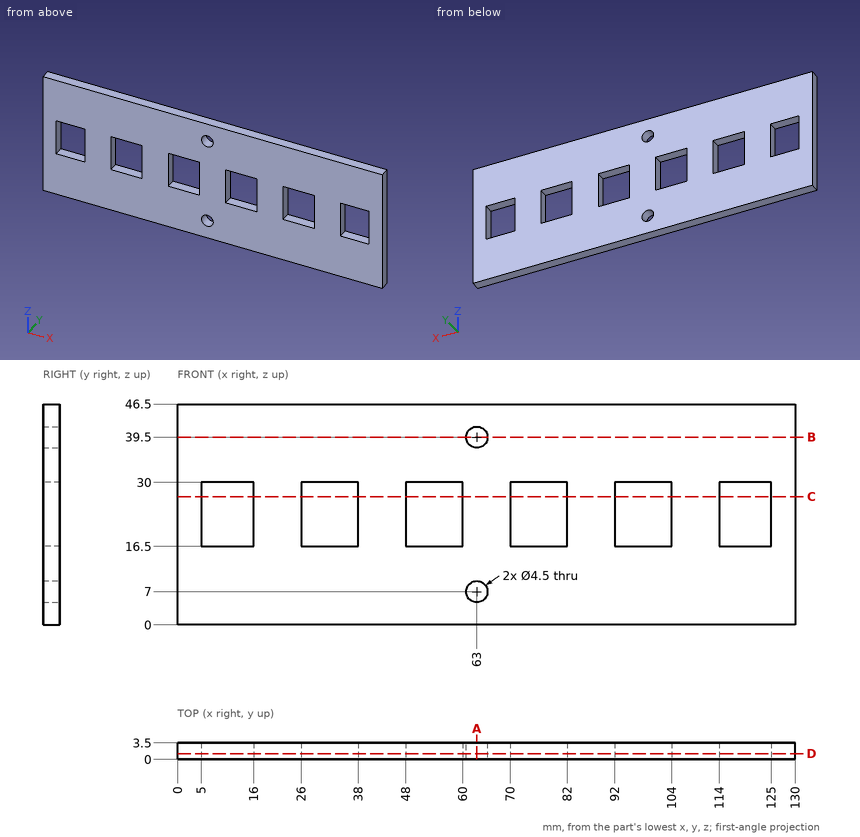
Could you check a few things on this drawing? It's one solid part, dimensions in mm from its lowest x, y, z. Give positions to 0.01 mm unless a question says otherwise; leave off trailing zeros. Order: outer loops, then holes, each group sorted by start corner. A loop starts at its lowest first (then second) coordinate and runs counter-clockwise, first axis right, second up. Notation, with made-up numbers: (-23, 74.25) - (19, 74.25) arc R29 cw to (19, 110.25) - close; hole circle Ø3 at (-30.5, 67). An arc over 180 degrees is marked (long way). Return JSON: item names as keys, results as strings. Group by question number.
Q1. Suppose I cut it at A-A, the plane x = 63. Please give me the cut outline in (y, z), and give its area (3 significant figures).
Q2. Will this pin go through, and if not, where does the flat tip stop? pin 1 Ø5 at (x, z) = (63, 39.5) entering from +Y.
Q3. Suppose I cut it at C-C, the plane z = 27. Please give me the cut outline in (x, y), and give its area (3 significant figures).
Q4. Suppose I cut it at B-B, the plane z = 39.5. Please give me the cut outline in (x, y).
Q5. Suppose I cut it at D-D, the plane y = 1.25. State how many separate pieces and enclosed holes the cut face has, and give its area (3 significant figures).
Q6. Please list where these lines run through material, in increasing order: line 1 along Z through (x, y) = (63, 1.4); line 2 along X through (y, z) = (2.2, 7); line 3 along Z through (x, y) = (119, 1.9). Write a range as [from, to].
Resolved:
{
 "1": {"outline": "(0, 0) - (3.5, 0) - (3.5, 4.75) - (0, 4.75) - close; (0, 9.25) - (3.5, 9.25) - (3.5, 37.25) - (0, 37.25) - close; (0, 41.75) - (3.5, 41.75) - (3.5, 46.5) - (0, 46.5) - close", "area": "131 mm2"},
 "2": {"pin 1": "stops at y = 3.5"},
 "3": {"outline": "(0, 0) - (5, 0) - (5, 3.5) - (0, 3.5) - close; (16, 0) - (26, 0) - (26, 3.5) - (16, 3.5) - close; (38, 0) - (48, 0) - (48, 3.5) - (38, 3.5) - close; (60, 0) - (70, 0) - (70, 3.5) - (60, 3.5) - close; (82, 0) - (92, 0) - (92, 3.5) - (82, 3.5) - close; (104, 0) - (114, 0) - (114, 3.5) - (104, 3.5) - close; (125, 0) - (130, 0) - (130, 3.5) - (125, 3.5) - close", "area": "210 mm2"},
 "4": {"outline": "(0, 0) - (60.75, 0) - (60.75, 3.5) - (0, 3.5) - close; (65.25, 0) - (130, 0) - (130, 3.5) - (65.25, 3.5) - close"},
 "5": {"separate pieces": "1", "enclosed holes": "8", "area": "5,070 mm2"},
 "6": {"line 1": "z = [0, 4.75], [9.25, 37.25], [41.75, 46.5]", "line 2": "x = [0, 60.75], [65.25, 130]", "line 3": "z = [0, 16.5], [30, 46.5]"}
}
